Read the model definition and answer for the solid it produces. Units are mm, in the model's axes. A direction names the side the tool comes from. Round coordinates to 2 decimals unless told otherwise and drop trailing zeros. Write each loop counter-clockwise with the first axis right and the second up, starting at its lowest first coordinate (ties: lowest second). Pieces come first, ordered by that corner, then holes.
from build123d import *

# Parameters (mm, degrees)
F0_W     = 50.8
F0_H     = 50.8
F1_DEPTH = 38.1
F2_SIZE  = 5.08


with BuildPart() as f1:
    # F0 (on Front) → F1 (new body)
    with BuildSketch(Plane.XZ):
        with BuildLine():
            ThreePointArc((-134.08614, -39.708438), (-130.366396, -48.688694), (-121.38614, -52.408438))
            Line((-121.38614, -52.408438), (-19.78614, -52.408438))
            ThreePointArc((-19.78614, -52.408438), (-7.08614, -39.708438), (5.61386, -52.408438))
            Line((5.61386, -52.408438), (107.21386, -52.408438))
            ThreePointArc((107.21386, -52.408438), (116.194116, -48.688694), (119.91386, -39.708438))
            Line((119.91386, -39.708438), (119.91386, 61.891562))
            ThreePointArc((119.91386, 61.891562), (116.194116, 70.871818), (107.21386, 74.591562))
            Line((107.21386, 74.591562), (5.61386, 74.591562))
            ThreePointArc((5.61386, 74.591562), (-7.08614, 61.891562), (-19.78614, 74.591562))
            Line((-19.78614, 74.591562), (-121.38614, 74.591562))
            ThreePointArc((-121.38614, 74.591562), (-130.366396, 70.871818), (-134.08614, 61.891562))
            Line((-134.08614, 61.891562), (-134.08614, -39.708438))
        make_face()
        with Locations((-7.08614, 11.091562)):
            Rectangle(F0_W, F0_H, mode=Mode.SUBTRACT)
    extrude(amount=F1_DEPTH)

    # F2
    f2_edges = [f1.edges().sort_by_distance(p)[0] for p in [
        (18.31386, -38.1, 11.091562),
        (-7.08614, -38.1, -14.308438),
        (-32.48614, -38.1, 11.091562),
        (-7.08614, -38.1, 36.491562),
        (-7.08614, 0, -14.308438),
        (-32.48614, 0, 11.091562),
        (18.31386, 0, 11.091562),
        (-7.08614, 0, 36.491562),
    ]]
    chamfer(f2_edges, length=F2_SIZE)


solid = f1.part
Q1. Determine the mould class of faces 4 (the flat face through (56, -19, -52.408)), 5 (the flat face through (-7.513, -2.504, -16.884)), 6 (the flat face through (-70, -19, 74.592)), 7 (the flat face through (-35.062, -2.504, 10.665)) for opening direction Z: pulls with the +Z half, pulls with the -Z half, needs draft (parallel to the pull), parting line crosses it, or undercut.
Verdict:
face 4: pulls with the -Z half
face 5: undercut
face 6: pulls with the +Z half
face 7: undercut
Q2. Section A-A (z = 66) is taken. Determine the outline of the cut face in (x, y), then the cut area to 3 significant figures.
Verdict:
outline: (-133.4, -38.1) - (-16.44, -38.1) - (-16.44, 0) - (-133.4, 0) - close; (2.27, -38.1) - (119.23, -38.1) - (119.23, 0) - (2.27, 0) - close
area: 8,910 mm2
Q3. Section C-C (z = -44) is taken. Determine the outline of the cut face in (x, y), then the cut area to 3 significant figures.
Verdict:
outline: (-133.34, -38.1) - (-16.6, -38.1) - (-16.6, 0) - (-133.34, 0) - close; (2.43, -38.1) - (119.17, -38.1) - (119.17, 0) - (2.43, 0) - close
area: 8,900 mm2
Q4. Straight lines are drawn through the part: probe 1 along Z at (x, y) = (-6.5, -23); probe 2 along X at (y, z) = (-32, 22); probe 3 along Z at (x, y) = (-25, -13.5). For each, find the intervals that lie inside material, in ascending order.
Verdict:
probe 1: z = -39.72 to -14.31, 36.49 to 61.91
probe 2: x = -134.09 to -32.49, 18.31 to 119.91
probe 3: z = -52.41 to -14.31, 36.49 to 74.59
Q5. A flat-ended cylindrical pin translates along its axis: pin 1 Ø8.5 at (x, y) = (-7, -13.5) entering from +Z. Find the tip coordinate at first contact, or state that the pin passes through.
Verdict:
pin 1: stops at z = 62.65
Q6. Section B-B (y = -14.5) is taken. Determine the outline of the cut face in (x, z), then the cut area to 3 significant figures.
Verdict:
outline: (-134.09, -39.71) arc R12.7 ccw to (-121.39, -52.41) - (-19.79, -52.41) arc R12.7 cw to (5.61, -52.41) - (107.21, -52.41) arc R12.7 ccw to (119.91, -39.71) - (119.91, 61.89) arc R12.7 ccw to (107.21, 74.59) - (5.61, 74.59) arc R12.7 cw to (-19.79, 74.59) - (-121.39, 74.59) arc R12.7 ccw to (-134.09, 61.89) - close; hole (-32.49, -14.31) - (18.31, -14.31) - (18.31, 36.49) - (-32.49, 36.49) - close
area: 29,000 mm2
Q7. Which of the six approach directions +Z, -Z, +X, -X, +Y, -Y give full straight-line access (tool end or side, diameter ignored) to faces 1 (the flat face through (-7, -19, -14.308)), 2 (the flat face through (20.889, -2.504, 10.665)), 3 (the flat face through (-7.51, -35.6, 39.07))?
Verdict:
face 1: +Y, -Y
face 2: +Y
face 3: -Y
